The figure shows three views and two pictorial views of one solid part (mm, origin at its lowest corner). Answer the questions. A direction names the side the tool comes from. Round coordinates to 2 decimals unless told otherwise and drop trailing zeros. Write each loop counter-clockwise with the first axis right and the second up, starting at its lowest first coordinate (ties: lowest second). Pieces come first, ordered by that corner, then holes.
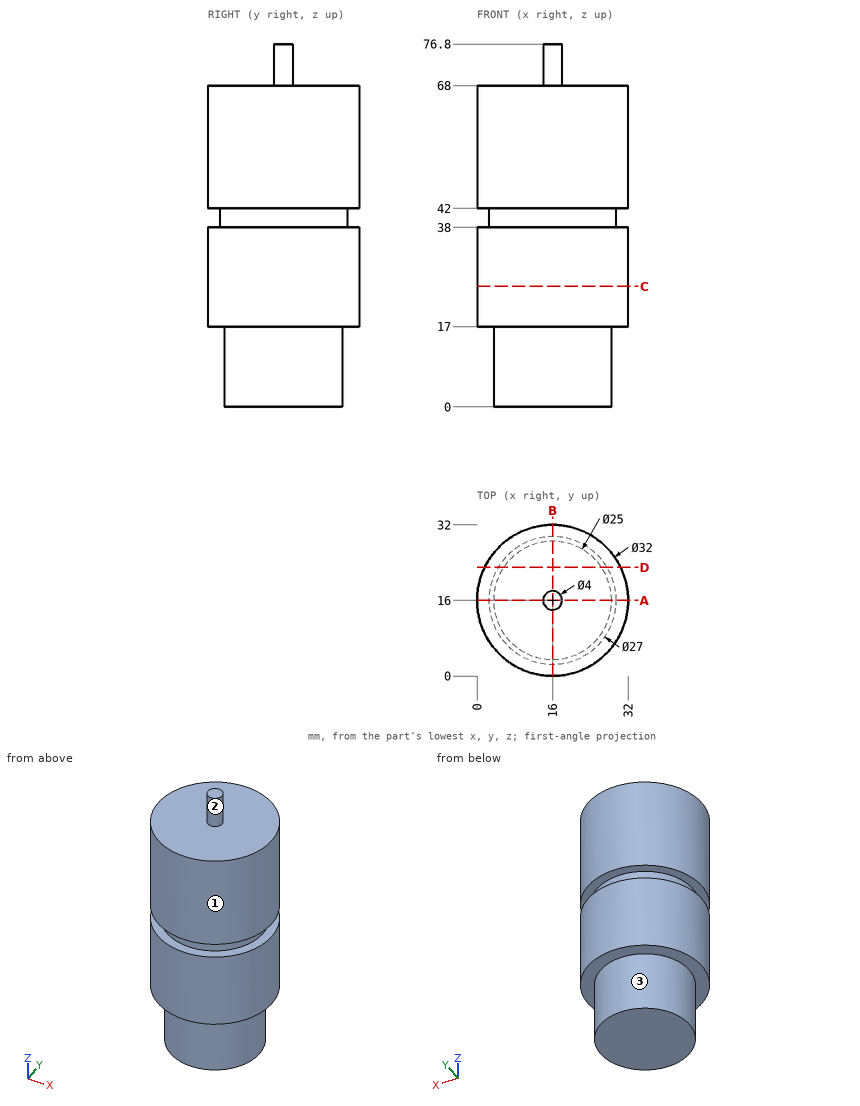
Q1. Section C-C (z = 25.5) is taken. Determine the outline of the cut face in (x, y), then the cut area to 3 significant figures.
Verdict:
outline: circle Ø32 at (16, 16)
area: 804 mm2
Q2. Which of the six approach directions +Z, -Z, +X, -X, +Y, -Y give full straight-line access (tool end or side, diameter ignored) to the marked faces 1, 2 and 3?
Verdict:
face 1: +Z, -Z
face 2: +Z
face 3: -Z
Q3. Section A-A (y = 16) is taken. Determine the outline of the cut face in (x, z).
Verdict:
outline: (0, 17) - (3.5, 17) - (3.5, 0) - (28.5, 0) - (28.5, 17) - (32, 17) - (32, 38) - (29.5, 38) - (29.5, 42) - (32, 42) - (32, 68) - (18, 68) - (18, 76.8) - (14, 76.8) - (14, 68) - (0, 68) - (0, 42) - (2.5, 42) - (2.5, 38) - (0, 38) - close
Q4. Flat-ended cylindrical pins translate along their axes: pin 1 Ø2 at (y, z) = (8, 13) entering from +X; pin 2 Ø16 at (x, y) = (11.5, 15) entering from -Z; pin 3 Ø6 at (y, z) = (9.5, 45) entering from +X; pin 4 Ø10 at (x, y) = (12, 4.5) entering from +Z. Find the tip coordinate at first contact, or state that the pin passes through.
Verdict:
pin 1: stops at x = 26.36
pin 2: stops at z = 0
pin 3: stops at x = 31.61
pin 4: stops at z = 68
Q5. Straight lines are drawn through the part: probe 1 along Z at (x, y) = (14, 23); probe 2 along Z at (x, y) = (10.5, 28); probe 3 along Y at (x, z) = (6, 37.5). For each, find the intervals that lie inside material, in ascending order.
Verdict:
probe 1: z = 0 to 68
probe 2: z = 17 to 68
probe 3: y = 3.51 to 28.49
Q6. Section D-D (y = 23) is taken. Determine the outline of the cut face in (x, z).
Verdict:
outline: (1.61, 17) - (5.64, 17) - (5.64, 0) - (26.36, 0) - (26.36, 17) - (30.39, 17) - (30.39, 38) - (27.54, 38) - (27.54, 42) - (30.39, 42) - (30.39, 68) - (1.61, 68) - (1.61, 42) - (4.46, 42) - (4.46, 38) - (1.61, 38) - close
